```python
from build123d import *

# Parameters (mm, degrees)
F0_R     = 0.75
F1_DEPTH = 20


with BuildPart() as f1:
    # F0 (on Top) → F1 (new body)
    with BuildSketch(Plane.XY):
        Polygon((-6.25, 8.5), (-8.5, 8.5), (-8.5, 6.25), (-8.5, 3.75), (-8.5, 1.25), (-8.5, -1.25), (-8.5, -3.75), (-8.5, -6.25), (-8.5, -8.5), (8.5, -8.5), (8.5, 8.5), (6.25, 8.5), (3.75, 8.5), (1.25, 8.5), (-1.25, 8.5), (-3.75, 8.5), align=None)
        with Locations((-6.293252, -6.249925)):
            Circle(F0_R, mode=Mode.SUBTRACT)
        with Locations((-3.793252, -6.249925)):
            Circle(F0_R, mode=Mode.SUBTRACT)
        with Locations((-1.293252, -6.249925)):
            Circle(F0_R, mode=Mode.SUBTRACT)
        with Locations((-6.284602, -3.74994)):
            Circle(F0_R, mode=Mode.SUBTRACT)
        with Locations((-6.275951, -1.249955)):
            Circle(F0_R, mode=Mode.SUBTRACT)
        with Locations((-3.784602, -3.74994)):
            Circle(F0_R, mode=Mode.SUBTRACT)
        with Locations((-1.284602, -3.74994)):
            Circle(F0_R, mode=Mode.SUBTRACT)
        with Locations((-3.775951, -1.249955)):
            Circle(F0_R, mode=Mode.SUBTRACT)
        with Locations((-1.275951, -1.249955)):
            Circle(F0_R, mode=Mode.SUBTRACT)
        with Locations((1.206748, -6.249925)):
            Circle(F0_R, mode=Mode.SUBTRACT)
        with Locations((3.706748, -6.249925)):
            Circle(F0_R, mode=Mode.SUBTRACT)
        with Locations((6.206748, -6.249925)):
            Circle(F0_R, mode=Mode.SUBTRACT)
        with Locations((1.215398, -3.74994)):
            Circle(F0_R, mode=Mode.SUBTRACT)
        with Locations((3.715398, -3.74994)):
            Circle(F0_R, mode=Mode.SUBTRACT)
        with Locations((1.224049, -1.249955)):
            Circle(F0_R, mode=Mode.SUBTRACT)
        with Locations((3.724049, -1.249955)):
            Circle(F0_R, mode=Mode.SUBTRACT)
        with Locations((6.215398, -3.74994)):
            Circle(F0_R, mode=Mode.SUBTRACT)
        with Locations((6.224049, -1.249955)):
            Circle(F0_R, mode=Mode.SUBTRACT)
        with Locations((-6.267301, 1.25003)):
            Circle(F0_R, mode=Mode.SUBTRACT)
        with Locations((-6.25865, 3.750015)):
            Circle(F0_R, mode=Mode.SUBTRACT)
        with Locations((-3.767301, 1.25003)):
            Circle(F0_R, mode=Mode.SUBTRACT)
        with Locations((-1.267301, 1.25003)):
            Circle(F0_R, mode=Mode.SUBTRACT)
        with Locations((-3.75865, 3.750015)):
            Circle(F0_R, mode=Mode.SUBTRACT)
        with Locations((-1.25865, 3.750015)):
            Circle(F0_R, mode=Mode.SUBTRACT)
        with Locations((-6.25, 6.25)):
            Circle(F0_R, mode=Mode.SUBTRACT)
        with Locations((-3.75, 6.25)):
            Circle(F0_R, mode=Mode.SUBTRACT)
        with Locations((-1.25, 6.25)):
            Circle(F0_R, mode=Mode.SUBTRACT)
        with Locations((1.232699, 1.25003)):
            Circle(F0_R, mode=Mode.SUBTRACT)
        with Locations((3.732699, 1.25003)):
            Circle(F0_R, mode=Mode.SUBTRACT)
        with Locations((1.24135, 3.750015)):
            Circle(F0_R, mode=Mode.SUBTRACT)
        with Locations((3.74135, 3.750015)):
            Circle(F0_R, mode=Mode.SUBTRACT)
        with Locations((6.232699, 1.25003)):
            Circle(F0_R, mode=Mode.SUBTRACT)
        with Locations((6.24135, 3.750015)):
            Circle(F0_R, mode=Mode.SUBTRACT)
        with Locations((1.25, 6.25)):
            Circle(F0_R, mode=Mode.SUBTRACT)
        with Locations((3.75, 6.25)):
            Circle(F0_R, mode=Mode.SUBTRACT)
        with Locations((6.25, 6.25)):
            Circle(F0_R, mode=Mode.SUBTRACT)
    extrude(amount=F1_DEPTH)


solid = f1.part
```
Could you check a few things on this model? Use its own coordinates, in mm. Give positions to 0.01 mm unless a question says otherwise; leave off trailing zeros. Order: outer loops, then holes, each group sorted by start corner. A loop starts at its lowest first (then second) coordinate and runs counter-clockwise, first axis right, second up.
Q1. Suppose I cut it at B-B, the plane z = 1.75. Count the separate pieces of the cut face and the enclosed holes in it, and give its area (3 significant figures).
Q2. We'd pull the mould along Y, two halves only. Please class faces 1 (the flat face through (0, 0, 20)), 2 (the cylindrical face through (-3.874, -0.506, 9.86)): +Y half, -Y half, draft (parallel to the pull), parting line (faces both ways), or undercut.
Q3. Suppose I cut it at A-A, the plane x = -6.25. Write out the boundary of the cut face in (y, z), and give its area (3 significant figures).
Solution:
1. separate pieces: 1
1. enclosed holes: 36
1. area: 225 mm2
2. face 1: draft
2. face 2: undercut
3. outline: (-8.5, 0) - (-7, 0) - (-7, 20) - (-8.5, 20) - close; (-5.5, 0) - (-4.5, 0) - (-4.5, 20) - (-5.5, 20) - close; (-3, 0) - (-2, 0) - (-2, 20) - (-3, 20) - close; (-0.5, 0) - (0.5, 0) - (0.5, 20) - (-0.5, 20) - close; (2, 0) - (3, 0) - (3, 20) - (2, 20) - close; (4.5, 0) - (5.5, 0) - (5.5, 20) - (4.5, 20) - close; (7, 0) - (8.5, 0) - (8.5, 20) - (7, 20) - close
3. area: 160 mm2
